Geometry check sheet. Reference: drawing and pictorial views, mm from the part's lowest x, y, z. A direction names the side the tool comes from. Coordinates: 2 decimals unless noted, no trailing zeros. Write each loop counter-clockwise with the first axis right and the second up, starting at its lowest first coordinate (ties: lowest second). Pieces come first, ordered by that corner, then holes. Notation, with made-up numbers: (49, -19) -> (57, -19) arc R9 cw to (57, -5) -> close; hole circle Ø8 at (-6.5, 2). An arc over 180 degrees is marked (long way). Use a Markdown table: item, result.
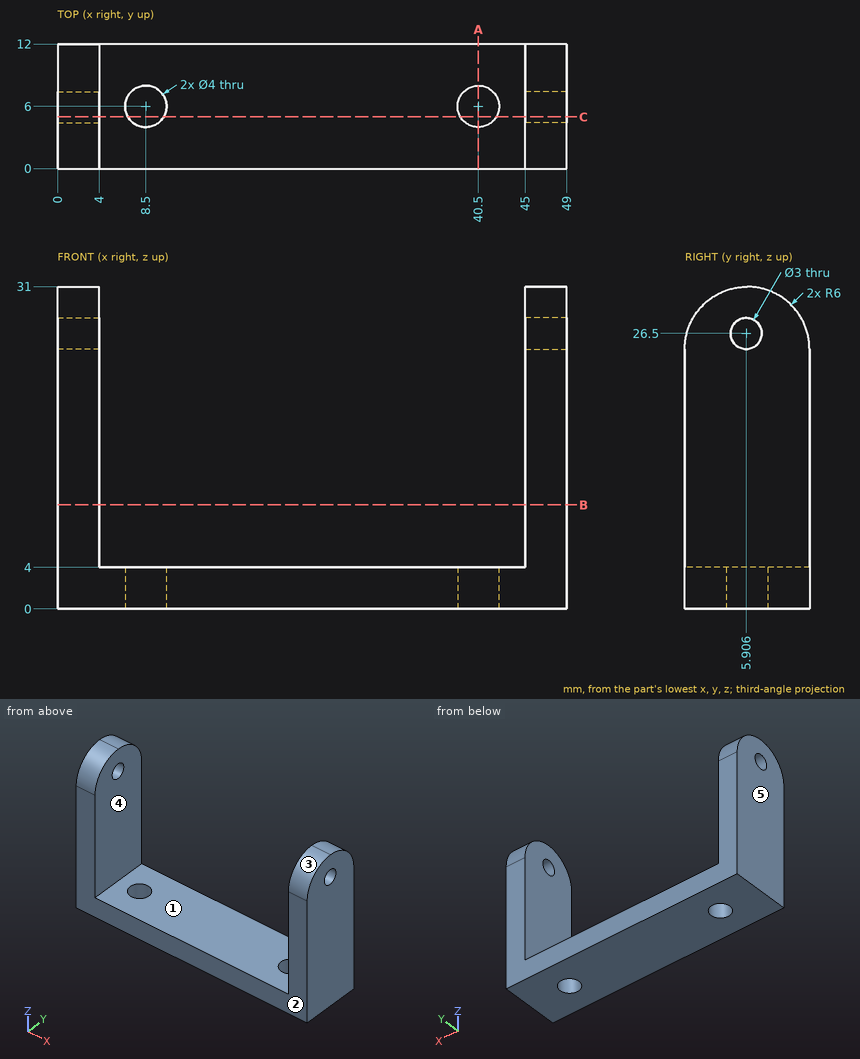
Item 1: Depth check by flat-ended pin: P1, Ø4, axis at y = 9.5, z = 5.5, coming from the -X side; P2, Ø5, axis at x = 40.5, y = 6, coming from the +Z side; P3, Ø2.5, axis at y = 5.91, z = 26.5, coming from the +X side. Enter the tip coordinate at first touch or a pass-through.
Answer block:
| item | result |
|---|---|
| P1 | stops at x = 0 |
| P2 | stops at z = 4 |
| P3 | passes through |
Item 2: Thickness scan on L1, parallel to X at y = 6, z = 1.35; L2, parallel to Y at x = 8.5, z = 2.4; L3, parallel to X at y = 9, z = 20. Record the ranges inside material, lowest first. Write a range as [from, to].
Answer block:
| item | result |
|---|---|
| L1 | x = [0, 6.5], [10.5, 38.5], [42.5, 49] |
| L2 | y = [0, 4], [8, 12] |
| L3 | x = [0, 4], [45, 49] |
Item 3: Tool access check on the marked faces 1 and 2. Record the directions out of +Z, -Z, +X, -X, +Y, -Y that give a thin tool (end or side, any length) a straight path to the whole face; none if there is none.
Answer block:
| item | result |
|---|---|
| face 1 | +Z, +Y, -Y |
| face 2 | +Z, -Z, +X, -X, -Y |
Item 4: Section check A-A on x = 40.5. Record the boundary of the cut face in (y, z), then the cut area to 3 significant figures.
Answer block:
| item | result |
|---|---|
| outline | (0, 0) -> (4, 0) -> (4, 4) -> (0, 4) -> close; (8, 0) -> (12, 0) -> (12, 4) -> (8, 4) -> close |
| area | 32.0 mm^2 |
Item 5: Section check C-C on y = 5. Record the boundary of the cut face in (x, z) (1 decimal).
Answer block:
| item | result |
|---|---|
| outline | (0, 0) -> (6.8, 0) -> (6.8, 4) -> (4, 4) -> (4, 25.3) -> (0, 25.3) -> close; (0, 27.7) -> (4, 27.7) -> (4, 30.9) -> (0, 30.9) -> close; (10.2, 0) -> (38.8, 0) -> (38.8, 4) -> (10.2, 4) -> close; (42.2, 0) -> (49, 0) -> (49, 25.3) -> (45, 25.3) -> (45, 4) -> (42.2, 4) -> close; (45, 27.7) -> (49, 27.7) -> (49, 30.9) -> (45, 30.9) -> close |
Item 6: Mould release check, pull along X, two halves, no side actions. Record for the marked faces 3, 4 and 5: +X half, -X half, draft (parallel to the pull), parting line (faces both ways), or undercut.
Answer block:
| item | result |
|---|---|
| face 3 | draft |
| face 4 | undercut |
| face 5 | -X half |
Item 7: Section check B-B on z = 10. Record the boundary of the cut face in (x, y).
Answer block:
| item | result |
|---|---|
| outline | (0, 0) -> (4, 0) -> (4, 12) -> (0, 12) -> close; (45, 0) -> (49, 0) -> (49, 12) -> (45, 12) -> close |
